from build123d import *

# Parameters (mm, degrees)
SKETCH1_W           = 58.1
SKETCH1_H           = 40.1
BOSS_EXTRUDE1_DEPTH = 10
SKETCH1_7_R         = 9.25
CUT_EXTRUDE1_DEPTH  = 10
SKETCH1_8_R         = 2.4
CUT_EXTRUDE2_DEPTH  = 10


with BuildPart() as part:
    # Sketch1 → Boss-Extrude1 (new body)
    with BuildSketch(Plane(origin=(0, 0, 0), x_dir=(1, 0, 0), z_dir=(0, 1, 0))):
        with Locations((40.179637899, 24.108385802)):
            Rectangle(SKETCH1_W, SKETCH1_H)
    extrude(amount=BOSS_EXTRUDE1_DEPTH)

    # Sketch1_7 → Cut-Extrude1 (cut)
    with BuildSketch(Plane(origin=(0, 0, 0), x_dir=(1, 0, 0), z_dir=(0, 1, 0))):
        with Locations(Location((31.329637899, 24.108385802, 0), (0, 0, 270))):
            Circle(SKETCH1_7_R)
    extrude(amount=CUT_EXTRUDE1_DEPTH, mode=Mode.SUBTRACT)

    # Sketch1_8 → Cut-Extrude2 (cut)
    with BuildSketch(Plane(origin=(0, 0, 0), x_dir=(1, 0, 0), z_dir=(0, 1, 0))):
        with Locations(Location((20.179637899, 38.108385802, 0), (0, 0, 270))):
            Circle(SKETCH1_8_R)
        with Locations(Location((60.179637899, 38.108385802, 0), (0, 0, 270))):
            Circle(SKETCH1_8_R)
        with Locations(Location((20.179637899, 10.108385802, 0), (0, 0, 270))):
            Circle(SKETCH1_8_R)
        with Locations(Location((60.179637899, 10.108385802, 0), (0, 0, 270))):
            Circle(SKETCH1_8_R)
    extrude(amount=CUT_EXTRUDE2_DEPTH, mode=Mode.SUBTRACT)


solid = part.part
The listing builds one solid part. Answer for the finished solid, in the listing's coordinates (mm). Coordinates: 2 decimals unless noted, no trailing zeros. Order: outer loops, then holes, each group sorted by start corner. A loop starts at its lowest first (then second) coordinate and runs counter-clockwise, first axis right, second up. Notation, with made-up numbers: M 78.5,22 L 93.5,22 A17 cw 93.5,53 Z; hole C 53,18 d9. An arc over 180 degrees is marked long. Use CSV: the item, a comma, the result in double quotes.
Q1. Section B-B (x = 24) is taken. Determine the outline of the cut face in (y, z), then the cut area to 3 significant figures.
Here are the results:
outline,"M 0,-44.16 L 10,-44.16 L 10,-29.75 L 0,-29.75 Z; M 0,-18.47 L 10,-18.47 L 10,-4.06 L 0,-4.06 Z"
area,"288 mm2"
Q2. Determine the mould class of faces 1 (the flat face through (11.13, 5, -24)), 2 (the cylindrical face through (37.581, 4.93, -30.926)), 3 (the flat face through (40, 5, -44.158)), 4 (the flat face through (69.23, 5, -24)) for opening direction X: pulls with the +X half, pulls with the -X half, needs draft (parallel to the pull), parting line crosses it, or undercut.
Here are the results:
face 1,"pulls with the -X half"
face 2,"undercut"
face 3,"needs draft"
face 4,"pulls with the +X half"
Q3. Section A-A (z = -30.5) is taken. Determine the outline of the cut face in (x, y), then the cut area to 3 significant figures.
Here are the results:
outline,"M 11.13,0 L 24.64,0 L 24.64,10 L 11.13,10 Z; M 38.02,0 L 69.23,0 L 69.23,10 L 38.02,10 Z"
area,"447 mm2"
Q4. Section D-D (x = 59) is taken. Determine the outline of the cut face in (y, z), then the cut area to 3 significant figures.
Here are the results:
outline,"M 0,-44.16 L 10,-44.16 L 10,-40.2 L 0,-40.2 Z; M 0,-36.02 L 10,-36.02 L 10,-12.2 L 0,-12.2 Z; M 0,-8.02 L 10,-8.02 L 10,-4.06 L 0,-4.06 Z"
area,"317 mm2"
Q5. Section C-C (z = -10.5) is taken. Determine the outline of the cut face in (x, y).
Here are the results:
outline,"M 11.13,0 L 17.81,0 L 17.81,10 L 11.13,10 Z; M 22.55,0 L 57.81,0 L 57.81,10 L 22.55,10 Z; M 62.55,0 L 69.23,0 L 69.23,10 L 62.55,10 Z"
Q6. Straight lines are drawn through the part: L1, parallel to Z at x = 21, y = 8; L2, parallel to X at y = 9.5, z = -37.5; L3, parallel to X at y = 7.25, z = -40. For each, find the intervals that lie inside material, in ascending order.
Here are the results:
L1,"-44.16 to -40.36, -35.85 to -12.36, -7.85 to -4.06"
L2,"11.13 to 17.86, 22.5 to 57.86, 62.5 to 69.23"
L3,"11.13 to 18.7, 21.66 to 58.7, 61.66 to 69.23"
